The listing builds one solid part. Answer for the finished solid, in the listing's coordinates (mm). A direction names the side the tool comes from. Coordinates: 2 decimals unless noted, no trailing zeros. Write each loop counter-clockwise with the first axis right and the second up, starting at its lowest first coordinate (ties: lowest second). Pieces come first, ordered by that corner, then holes.
from build123d import *

# Parameters (mm, degrees)
SKETCH1_R           = 38.1
BOSS_EXTRUDE1_DEPTH = 5
SKETCH5_R           = 1.75
CUT_EXTRUDE5_DEPTH  = 3
SKETCH6_R           = 2.5
CUT_EXTRUDE6_DEPTH  = 3
SKETCH7_R           = 6.25
CUT_EXTRUDE7_DEPTH  = 2.5
SKETCH8_R           = 5
CUT_EXTRUDE10_DEPTH = 55.113029854


with BuildPart() as part:
    # Sketch1 → Boss-Extrude1 (new body)
    with BuildSketch(Plane(origin=(0, 0, 0), x_dir=(1, 0, 0), z_dir=(0, 1, 0))):
        with Locations(Location((0, 0, 0), (0, 0, 270))):
            Circle(SKETCH1_R)
    extrude(amount=BOSS_EXTRUDE1_DEPTH)

    # Sketch5 → Cut-Extrude5 (cut)
    with BuildSketch(Plane(origin=(0, 5, 0), x_dir=(1, 0, 0), z_dir=(0, 1, 0))):
        with Locations(Location((21.213203436, 21.213203436, 0), (0, 0, 270))):
            Circle(SKETCH5_R)
        with Locations(Location((-21.213203436, 21.213203436, 0), (0, 0, 270))):
            Circle(SKETCH5_R)
        with Locations(Location((-21.213203436, -21.213203436, 0), (0, 0, 270))):
            Circle(SKETCH5_R)
        with Locations(Location((21.213203436, -21.213203436, 0), (0, 0, 270))):
            Circle(SKETCH5_R)
    extrude(amount=-CUT_EXTRUDE5_DEPTH, mode=Mode.SUBTRACT)

    # Sketch6 → Cut-Extrude6 (cut)
    with BuildSketch(Plane.XZ):
        with Locations(Location((0, -33.1, 0), (0, 0, 270))):
            Circle(SKETCH6_R)
        with Locations(Location((33.1, 0, 0), (0, 0, 270))):
            Circle(SKETCH6_R)
        with Locations(Location((0, 33.1, 0), (0, 0, 270))):
            Circle(SKETCH6_R)
        with Locations(Location((-33.1, 0, 0), (0, 0, 270))):
            Circle(SKETCH6_R)
    extrude(amount=-CUT_EXTRUDE6_DEPTH, mode=Mode.SUBTRACT)

    # Sketch7 → Cut-Extrude7 (cut)
    with BuildSketch(Plane(origin=(0, 5, 0), x_dir=(1, 0, 0), z_dir=(0, 1, 0))):
        with Locations(Location((0, 0, 0), (0, 0, 270))):
            Circle(SKETCH7_R)
    extrude(amount=-CUT_EXTRUDE7_DEPTH, mode=Mode.SUBTRACT)

    # Sketch8 → Cut-Extrude10 (cut, through all)
    with BuildSketch(Plane(origin=(0, 5, 0), x_dir=(1, 0, 0), z_dir=(0, 1, 0))):
        with Locations(Location((0, 0, 0), (0, 0, 270))):
            Circle(SKETCH8_R)
    extrude(amount=-CUT_EXTRUDE10_DEPTH, mode=Mode.SUBTRACT)


solid = part.part
Q1. The part is cut by section D-D, the plane x = -33.1. Write down the section's boundary in (y, z), then the cut area to 3 significant figures.
Answers below:
outline: (0, -18.87) - (5, -18.87) - (5, 18.87) - (0, 18.87) - (0, 2.5) - (3, 2.5) - (3, -2.5) - (0, -2.5) - close
area: 174 mm2
Q2. Determine the mould class of faces 1 (the face through (1, 5, 8)), 2 (the face through (-23.183, 2.465, -30.235)), 3 (the face through (21, 2, 21)) for opening direction X: released by +X, released by -X, zero draft, split by the parting line, or undercut.
Answers below:
face 1: zero draft
face 2: split by the parting line
face 3: undercut
Q3. The part is cut by section A-A, the plane x = 0. Write down the section's boundary in (y, z).
Answers below:
outline: (0, -38.1) - (5, -38.1) - (5, -6.25) - (2.5, -6.25) - (2.5, -5) - (0, -5) - (0, -30.6) - (3, -30.6) - (3, -35.6) - (0, -35.6) - close; (0, 5) - (2.5, 5) - (2.5, 6.25) - (5, 6.25) - (5, 38.1) - (0, 38.1) - (0, 35.6) - (3, 35.6) - (3, 30.6) - (0, 30.6) - close
Q4. Find the intervals of material crossed by probe 1 along X at (y, z) = (1, 0); probe 2 along Z at (x, y) = (-20.5, 2.7); probe 3 along Z at (x, y) = (-0.5, 3.75), in increasing order.
Answers below:
probe 1: x = -38.1 to -35.6, -30.6 to -5, 5 to 30.6, 35.6 to 38.1
probe 2: z = -32.11 to -22.81, -19.62 to 19.62, 22.81 to 32.11
probe 3: z = -38.1 to -6.23, 6.23 to 38.1
Q5. The part is cut by section B-B, the plane z = 0. Write down the section's boundary in (x, y), then the cut area to 3 significant figures.
Answers below:
outline: (-38.1, 0) - (-35.6, 0) - (-35.6, 3) - (-30.6, 3) - (-30.6, 0) - (-5, 0) - (-5, 2.5) - (-6.25, 2.5) - (-6.25, 5) - (-38.1, 5) - close; (5, 0) - (30.6, 0) - (30.6, 3) - (35.6, 3) - (35.6, 0) - (38.1, 0) - (38.1, 5) - (6.25, 5) - (6.25, 2.5) - (5, 2.5) - close
area: 295 mm2
Q6. Given pin 1 (2 mm diameter, centred on y = 3.5, z = -10.5, fed in from -X); pin 2 (3 mm diameter, centred on x = -18, z = 24, fed in from -Y); pin 3 (8 mm diameter, centred on x = 0, z = 0, fed in from -Y); pin 4 (2.5 mm diameter, centred on x = 0, z = 33, fed in from -Y), each flat-ended and moving along its own axis, determine where each tip first touches the part or whether it passes through.
Answers below:
pin 1: stops at x = -36.9
pin 2: stops at y = 0
pin 3: passes through
pin 4: stops at y = 3
Q7. The part is cut by section C-C, the plane y = 1.25. Write down the section's boundary in (x, z).
Answers below:
outline: circle Ø76.2 at (0, 0); hole circle Ø5 at (-33.1, 0); hole circle Ø10 at (0, 0); hole circle Ø5 at (0, -33.1); hole circle Ø5 at (0, 33.1); hole circle Ø5 at (33.1, 0)
Q8. Which of the six approach directions +Z, -Z, +X, -X, +Y, -Y give full straight-line access (tool end or side, diameter ignored) to faces 4 (the face through (-4.88, 1.27, -1.08)), 5 (the face through (-0.96, 1.48, 30.79)), 6 (the face through (22.69, 3.52, 22.15))?
Answers below:
face 4: +Y, -Y
face 5: -Y
face 6: +Y
